For this review, take the finished solid that the model builds, in its own axes (mm). Face numbers are marked on the shaded views. A direction names the side the tool comes from. Coordinates: 2 decimals unless noted, no trailing zeros. Order: outer loops, then holes, each group sorted by start corner. A loop starts at its lowest first (then second) coordinate and runs counter-clockwise, first axis right, second up. Notation, with made-up numbers: (2, -26.75) -> (20, -26.75) arc R26 cw to (20, 6.25) -> close; hole circle Ø7 at (36.25, -20.5). An arc over 180 degrees is marked (long way). Write item = value, one per line. Start each with the question number.
1) Wall thickness on probe 1 along Z at (x, y) = (-61, 215.5); probe 2 along Z at (x, y) = (-61.05, 192.25); probe 3 along X at (y, z) = (188, -42.5): over which ranges is each line inside the solid? List them lowest first. Write a range as [from, to].
2) Machinability: for the marked faces 1 and 2, which of the approach directions +Z, -Z, +X, -X, +Y, -Y give a long, thin tool a straight path to every point of the face, cutting with its end or side? Answer none if there is none.
3) Insertion check: pin 1 Ø3 at (y, z) = (192.25, -13.08) entering from -X; pin 2 Ø6.5 at (x, y) = (-48.5, 208) entering from -Z; pin 3 Ø3 at (y, z) = (198, -44.5) entering from +X. Each pin has a flat end and moves straight along its axis. Give the tip position at first contact, or say it passes through.
4) Consider section D-D on x = -61. Give the boundary of the cut face in (y, z), and give its area (3 significant figures).
5) Consider section C-C on x = -48. Give the boundary of the cut face in (y, z).
6) Consider section B-B on z = -41.3. Give the boundary of the cut face in (x, y), and give its area (3 significant figures).
7) Consider section A-A on y = 207.75. Give the boundary of the cut face in (x, z), and give its area (3 significant figures).
from build123d import *

# Parameters (mm, degrees)
SKETCH_1_W                  = 40
SKETCH_1_H                  = 45
EXTRUDE_1_DEPTH             = 25
SKETCH_2_W                  = 22
SKETCH_2_H                  = 50
CUT_EXTRUDE_1_DEPTH         = 90.827612681
SKETCH_3_R                  = 3
CUT_EXTRUDE_2_DEPTH         = 227.991189256
HOLE_WIZARD_4_2_4_2_1_D     = 4.2
HOLE_WIZARD_3_2_3_2_1_D     = 3.2
HOLE_WIZARD_3_2_3_2_1_DEPTH = 25


with BuildPart() as part:
    # 草图1 → 凸台-拉伸1 (new body)
    with BuildSketch(Plane(origin=(-63, 0, 0), x_dir=(0, -1, 0), z_dir=(-1, 0, 0))):
        with Locations((-200, -27.5)):
            Rectangle(SKETCH_1_W, SKETCH_1_H)
    extrude(amount=-EXTRUDE_1_DEPTH)

    # 草图2 → 切除-拉伸1 (cut, through all)
    with BuildSketch(Plane(origin=(0, 220, 0), x_dir=(-1, 0, 0), z_dir=(0, 1, 0))):
        with Locations((49, -33)):
            Rectangle(SKETCH_2_W, SKETCH_2_H)
    extrude(amount=-CUT_EXTRUDE_1_DEPTH, mode=Mode.SUBTRACT)

    # 草图3 → 切除-拉伸2 (cut, through all)
    with BuildSketch(Plane.ZY.offset(63)):
        with Locations(Location((-41.3, 200, 0), (0, 0, 270))):
            Circle(SKETCH_3_R)
    extrude(amount=-CUT_EXTRUDE_2_DEPTH, mode=Mode.SUBTRACT)

    # Ø4.2 (4.2) 直径孔1 (through all)
    with Locations(Plane(origin=(0, 0, -8), x_dir=(-1, 0, 0), z_dir=(0, 0, -1))):
        with Locations((48, 215), (48, 185)):
            Hole(HOLE_WIZARD_4_2_4_2_1_D / 2)

    # Ø3.2 (3.2) 直径孔1
    with Locations(Plane.ZY.offset(63)):
        with Locations((-26.5, 215.5), (-26.5, 184.5), (-13.076606241, 207.75), (-13.076606241, 192.25)):
            Hole(HOLE_WIZARD_3_2_3_2_1_D / 2, depth=HOLE_WIZARD_3_2_3_2_1_DEPTH)


solid = part.part
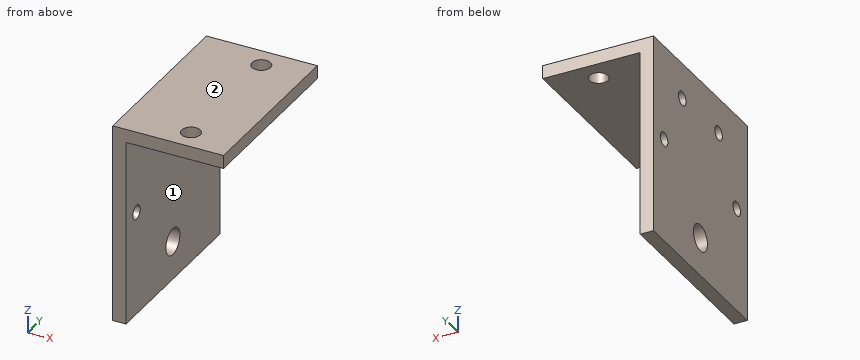
Answer sheet:
q1.probe_1 = [-50, -28.1], [-24.9, -5]
q1.probe_2 = [-50, -14.68], [-11.48, -5]
q1.probe_3 = [-63, -60]
q2.face_1 = -Z, +X, +Y, -Y
q2.face_2 = +Z, +X, -X, +Y, -Y
q3.pin_1 = through
q3.pin_2 = -8
q3.pin_3 = -60
q4.outline = (180, -50) -> (220, -50) -> (220, -5) -> (180, -5) -> close; hole circle Ø3.2 at (184.5, -26.5); hole circle Ø3.2 at (192.25, -13.08); hole circle Ø6 at (200, -41.3); hole circle Ø3.2 at (207.75, -13.08); hole circle Ø3.2 at (215.5, -26.5)
q4.area = 1,740 mm2
q5.outline = (180, -8) -> (182.9, -8) -> (182.9, -5) -> (180, -5) -> close; (187.1, -8) -> (212.9, -8) -> (212.9, -5) -> (187.1, -5) -> close; (217.1, -8) -> (220, -8) -> (220, -5) -> (217.1, -5) -> close
q6.outline = (-63, 180) -> (-60, 180) -> (-60, 197) -> (-63, 197) -> close; (-63, 203) -> (-60, 203) -> (-60, 220) -> (-63, 220) -> close
q6.area = 102 mm2
q7.outline = (-63, -50) -> (-60, -50) -> (-60, -14.68) -> (-63, -14.68) -> close; (-63, -11.48) -> (-60, -11.48) -> (-60, -8) -> (-38, -8) -> (-38, -5) -> (-63, -5) -> close
q7.area = 191 mm2
